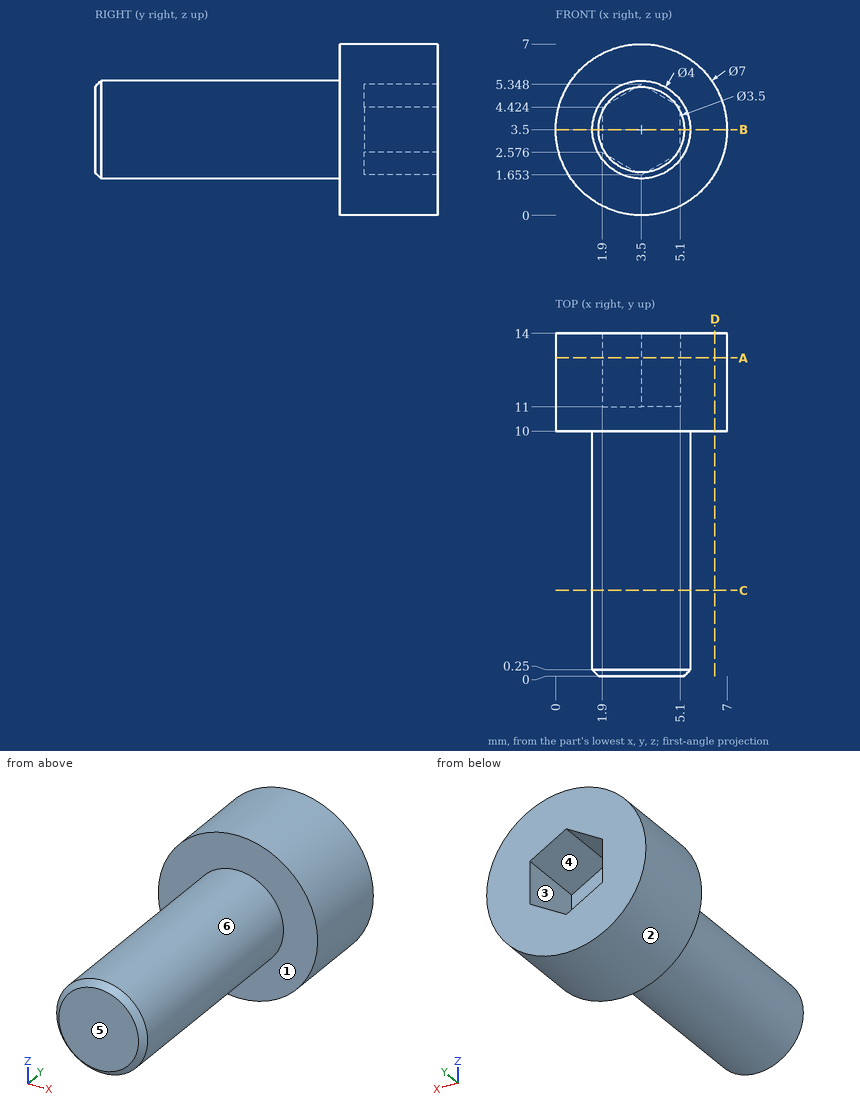
Print and shaded views of the part. All mm, measured from the part's lowest x, y and z. A direction names the side the tool comes from. Round coordinates to 2 decimals unless told otherwise and drop trailing zeros. Write each loop counter-clockwise with the first axis right and the second up, starting at its lowest first coordinate (ties: lowest second). Pieces come first, ordered by that corner, then holes. Notation, with made-up numbers: M 32,-32.5 L 80,-32.5 A27 ccw 80,-16.5 Z; hole C 43,45 d10. An arc over 180 degrees is marked long. Use a Markdown table: item, result. Add a question column.
1. Drill centre lines: probe 1 along Y at (x, z) = (4, 4.5); probe 2 along Y at (x, z) = (1, 2.5); probe 3 along Z at (x, y) = (3, 11.75) (1 decimal). Where is each one in solid material? Low to high.
2. 3-axis set-ups, long thin cutter, end or side, ignore diameter. For the marked faces 4, 5 and 6: which of +Z, -Z, +X, -X, +Y, -Y reach the whole face in a straight line?
3. Slice it at D-D on x = 6.5. Give the cut face in (y, z), then the cut area to 3 significant figures.
4. Slice it at B-B on z = 3.5. Give the cut face in (x, y).
5. Slice it at A-A on y = 13. Give the cut face in (x, z), then the cut area to 3 significant figures.
6. Slice it at C-C on y = 3.5. Give the cut face in (x, z).
7. Pull direction Z, two halves, no side cores. Call the marked faces 1, 2 and 3: released by +Z, released by -Z, zero draft, split by the parting line, or undercut.
8. Flat gauge pins, fed straight in: P1, Ø1, axis at x = 4.5, y = 10, coming from the +Z side; P2, Ø2, axis at x = 3, z = 2, coming from the +Y side. Where does each tip first touch, or does it go through?
Reply:
| question | item | result |
|---|---|---|
| 1 | probe 1 | y = 0 to 11 |
| 1 | probe 2 | y = 10 to 14 |
| 1 | probe 3 | z = 0 to 1.9, 5.1 to 7 |
| 2 | face 4 | +Y |
| 2 | face 5 | +Z, -Z, +X, -X, -Y |
| 2 | face 6 | -Y |
| 3 | outline | M 10,1.7 L 14,1.7 L 14,5.3 L 10,5.3 Z |
| 3 | area | 14.4 mm^2 |
| 4 | outline | M 0,10 L 1.5,10 L 1.5,0.25 L 1.75,0 L 5.25,0 L 5.5,0.25 L 5.5,10 L 7,10 L 7,14 L 5.1,14 L 5.1,11 L 1.9,11 L 1.9,14 L 0,14 Z |
| 5 | outline | C 3.5,3.5 d7; hole M 1.9,2.58 L 3.5,1.65 L 5.1,2.58 L 5.1,4.42 L 3.5,5.35 L 1.9,4.42 Z |
| 5 | area | 29.6 mm^2 |
| 6 | outline | C 3.5,3.5 d4 |
| 7 | face 1 | zero draft |
| 7 | face 2 | split by the parting line |
| 7 | face 3 | undercut |
| 8 | P1 | stops at z = 6.96 |
| 8 | P2 | stops at y = 14 |
